Read the model definition and answer for the solid it produces. Units are mm, in the model's axes. A direction names the side the tool comes from. Round coordinates to 2 decimals unless told otherwise and drop trailing zeros. Order: outer loops, then holes, each group sorted by start corner. A loop starts at its lowest first (then second) coordinate and runs counter-clockwise, first axis right, second up. Notation, with made-up numbers: (31, -29.75) -> (38, -29.75) arc R22 ccw to (38, -13.75) -> close; hole circle Ø4 at (2, -18.5). An arc over 180 degrees is marked (long way). Use a Markdown table: item, result. Add a question column.
1. Section C-C, the plane x = 3.5 is taken. Give the vertices of the cut face in (y, z), then the cut area to 3 significant figures.
2. Section B-B, the plane z = -4.5 is taken. Give the vertices of the cut face in (x, y).
3. Section D-D, the plane y = 10.25 is taken. Give the vertices of the cut face in (x, z).
4. For faces 1 (the face through (0, 18, 0)), 2 (the face through (-5, 6, -5)), determine the directions among +Z, -Z, +X, -X, +Y, -Y from which every point of the face is accessible in a straight line to the end or side of a thin tool.
5. Section A-A, the plane y = 3.5 is taken. Give the vertices of the cut face in (x, z).
6. Consider L1, parallel to Y at x = 3.25, z = -2.5; L2, parallel to Y at x = 6.5, z = -5.75; L3, parallel to Z at x = 5, y = 5.5. Determine where each line is inside the solid, lowest interval first. Write a range as [from, to].
7. Given pin 1 (8 mm diameter, centred on x = 6.5, z = 5, fed in from +Y); pin 2 (10 mm diameter, centred on x = 7, z = 1.5, fed in from +Y); pin 3 (8 mm diameter, centred on x = -6, y = 15.5, fed in from -Z); pin 4 (1 mm diameter, centred on y = 7, z = -4.5, fed in from +X), each flat-ended and moving along its own axis, determine where each tip first touches the part or whether it passes through.
Autodesk Inventor part; units mm, degrees
ref_plane "Work Plane1" through (0, 18, 0) normal (0, 1, 0) x (1, 0, 0)
ref_plane "YZ Plane" through (0, 0, 0) normal (1, 0, 0) x (0, 1, 0)
ref_plane "XZ Plane" through (0, 0, 0) normal (0, 1, 0) x (-1, 0, 0)
sketch "Sketch1" plane through (0, 0, 0) normal (0, 1, 0) x (-1, 0, 0)
  circle A0 centre (0, 0) radius 11
  dimension "d0" = 22
extrude "Extrusion1" add sketch "Sketch1" along normal blind 6
sketch "Sketch2" plane through (0, 6, 0) normal (0, 1, 0) x (1, 0, 0)
  circle A0 centre (0, 0) radius 6
  dimension "d3" = 12
extrude "Extrusion2" add sketch "Sketch2" along normal blind 5
sketch "Sketch3" plane through (0, 11, 0) normal (0, 1, 0) x (1, 0, 0)
  line L0 (-3, -3) -> (3, -3)
  line L1 (3, -3) -> (3, 3)
  line L2 (3, 3) -> (-3, 3)
  line L3 (-3, 3) -> (-3, -3)
  point P0 (0, 0)
  dimension "d6" = 6
  dimension "d7" = 6
ref_plane "Work Plane1" through (0, 18, 0) normal (0, 1, 0) x (1, 0, 0)
sketch "Sketch4" plane through (0, 18, 0) normal (0, 1, 0) x (1, 0, 0)
  line L0 (-2.5, -2.5) -> (2.5, -2.5)
  line L1 (2.5, -2.5) -> (2.5, 2.5)
  line L2 (2.5, 2.5) -> (-2.5, 2.5)
  line L3 (-2.5, 2.5) -> (-2.5, -2.5)
  point P0 (0, 0)
  dimension "d9" = 5
  dimension "d10" = 5
loft "Loft1" add profiles "Sketch3", "Sketch4"
properties part number "Driveshaft coupling end"
Verdict:
| question | item | result |
|---|---|---|
| 1 | outline | (0, -10.43) -> (6, -10.43) -> (6, -4.87) -> (11, -4.87) -> (11, 4.87) -> (6, 4.87) -> (6, 10.43) -> (0, 10.43) -> close |
| 1 | area | 174 mm2 |
| 2 | outline | (-10.04, 0) -> (10.04, 0) -> (10.04, 6) -> (3.97, 6) -> (3.97, 11) -> (-3.97, 11) -> (-3.97, 6) -> (-10.04, 6) -> close |
| 3 | outline | circle Ø12 at (0, 0) |
| 4 | face 1 | +Z, -Z, +X, -X, +Y |
| 4 | face 2 | +Y |
| 5 | outline | circle Ø22 at (0, 0) |
| 6 | L1 | y = [0, 11] |
| 6 | L2 | y = [0, 6] |
| 6 | L3 | z = [-9.8, 9.8] |
| 7 | pin 1 | stops at y = 11 |
| 7 | pin 2 | stops at y = 18 |
| 7 | pin 3 | stops at z = -2.86 |
| 7 | pin 4 | stops at x = 4.47 |
